The listing builds one solid part. Answer for the finished solid, in the listing's coordinates (mm). Round coordinates to 2 decimals unless told otherwise and drop trailing zeros. Loops run counter-clockwise (first coordinate to the right, second up) from the corner with the lowest first, then second, coordinate; pieces in that order, holes last. Notation, with made-up numbers: (42, -20.75) -> (86, -20.75) arc R30 cw to (86, 1.25) -> close; hole circle Ø2 at (63, -0.75). An arc over 180 degrees is marked (long way). Write each question's results on one line, items separated by ' | '. Start each with the question number.
from build123d import *

# Parameters (mm, degrees)
BOX002_W              = 14
BOX002_H              = 16
BOX002_DEPTH          = 8
SKETCH003_R           = 2.5
POCKET001002002_DEPTH = 8
SKETCH004_R           = 2.5
SKETCH004_R_2         = 1.05
POCKET001002003_DEPTH = 14


with BuildPart() as part:
    # Box002 → Box002 (new body)
    with BuildSketch(Plane(origin=(-4.5, -12, -16), x_dir=(1, 0, 0), z_dir=(0, 0, 1))):
        with Locations((7, 8)):
            Rectangle(BOX002_W, BOX002_H)
    extrude(amount=BOX002_DEPTH)

    # Sketch003 → Pocket001002002 (cut)
    with BuildSketch(Plane(origin=(-4.5, -12, -8), x_dir=(1, 0, 0), z_dir=(0, 0, 1))):
        with Locations((4.5, 12)):
            Circle(SKETCH003_R)
    extrude(amount=-POCKET001002002_DEPTH, mode=Mode.SUBTRACT)

    # Sketch004 → Pocket001002003 (cut)
    with BuildSketch(Plane(origin=(9.5, -12, -16), x_dir=(0, 1, 0), z_dir=(1, 0, 0))):
        with Locations((4, 4)):
            Circle(SKETCH004_R)
        with Locations((7.75, 2.15)):
            Circle(SKETCH004_R_2)
    extrude(amount=-POCKET001002003_DEPTH, mode=Mode.SUBTRACT)


solid = part.part
Item 1: The part is cut by section B-B, the plane y = -1.5. Give the vertices of the cut face in (x, z), plus the area to 3 significant figures.
Item 2: Straight lines are drawn through the part: L1, parallel to Y at x = 0, z = -11; L2, parallel to Z at x = 2.75, y = -8; L3, parallel to Y at x = 2, z = -15.25. For each, find the intervals that lie inside material, in ascending order. Write a range as [from, to].
Item 3: The part is cut by section D-D, the plane x = -3. Give the vertices of the cut face in (y, z).
Item 4: The part is cut by section C-C, the plane x = 0. Give the vertices of the cut face in (y, z).
Item 5: The part is cut by section A-A, the plane z = -10. Give the vertices of the cut face in (x, y).
Item 6: This flat-tipped pin is pushed along its axis until it touches: pin 1 Ø1.9 at (y, z) = (-4.25, -13.85) entering from -X. Where does it stop, or does it pass through?
Item 7: Determine the mould class of faces 1 (the cylindrical face through (-0.54, -2.44, -11.94)), 2 (the flat face through (2, -12, -12)), 3 (the flat face through (-4.5, -4, -12)), 4 (the flat face through (2, 4, -12)) for opening direction Y: +Y half, -Y half, draft (parallel to the pull), parting line (faces both ways), or undercut.
Report:
1) outline: (-4.5, -16) -> (-2, -16) -> (-2, -8) -> (-4.5, -8) -> close; (2, -16) -> (9.5, -16) -> (9.5, -8) -> (2, -8) -> close | area: 80.0 mm2
2) L1: y = [-12, -10.29], [-5.71, -2.5], [2.5, 4] | L2: z = [-16, -14.5], [-9.5, -8] | L3: y = [-12, -1.5], [1.5, 4]
3) outline: (-12, -16) -> (4, -16) -> (4, -8) -> (-12, -8) -> close; hole circle Ø5 at (-8, -12); hole circle Ø2.1 at (-4.25, -13.85)
4) outline: (-12, -16) -> (-2.5, -16) -> (-2.5, -8) -> (-12, -8) -> close; (2.5, -16) -> (4, -16) -> (4, -8) -> (2.5, -8) -> close; hole circle Ø5 at (-8, -12); hole circle Ø2.1 at (-4.25, -13.85)
5) outline: (-4.5, -12) -> (9.5, -12) -> (9.5, -9.5) -> (-4.5, -9.5) -> close; (-4.5, -6.5) -> (9.5, -6.5) -> (9.5, 4) -> (-4.5, 4) -> close; hole circle Ø5 at (0, 0)
6) pin 1: passes through
7) face 1: undercut | face 2: -Y half | face 3: draft | face 4: +Y half
